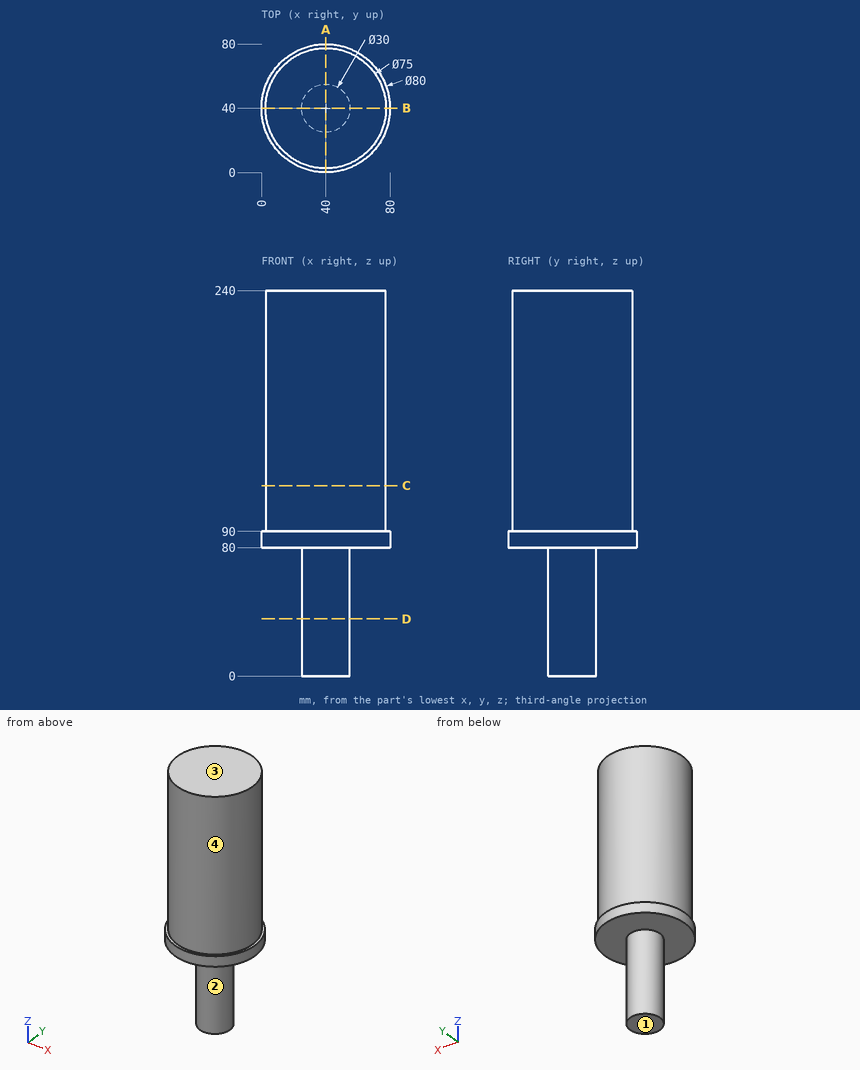
Geometry check sheet. Reference: drawing and pictorial views, mm from the part's lowest x, y, z. A direction names the side the tool comes from. Round coordinates to 2 decimals unless told otherwise and drop trailing zeros. Write each loop counter-clockwise with the first axis right and the second up, starting at its lowest first coordinate (ties: lowest second). Pieces come first, ordered by that corner, then holes.
(1) Section check D-D (z = 35.5). Enter the section's corners in (x, y), plus the area to 3 significant figures.
Returned:
outline: circle Ø30 at (40, 40)
area: 707 mm2
(2) Material ranges on line 1 (Z direction, x = 10, y = 33.5); line 2 (Y direction, x = 41.5, z = 188.5); line 3 (Z direction, x = 63, y = 9.5), recorded low to high.
Returned:
line 1: z = 80 to 240
line 2: y = 2.53 to 77.47
line 3: z = 80 to 90
(3) Section check A-A (x = 40). Enter the section's corners in (y, z), plus the area to 4 significant figures.
Returned:
outline: (0, 80) - (25, 80) - (25, 0) - (55, 0) - (55, 80) - (80, 80) - (80, 90) - (77.5, 90) - (77.5, 240) - (2.5, 240) - (2.5, 90) - (0, 90) - close
area: 14,450 mm2
(4) Mould release check, pull along Y, two halves, no side actions. Record for the marked faces 3 and 4: pulls with the +Y half, pulls with the -Y half, needs draft (parallel to the pull), parting line crosses it, or undercut.
Returned:
face 3: needs draft
face 4: parting line crosses it
(5) Section check C-C (z = 118.5). Enter the section's corners in (x, y), plus the area to 3 significant figures.
Returned:
outline: circle Ø75 at (40, 40)
area: 4,420 mm2
(6) Access from +Z, -Z, +X, -X, +Y, -Y to the whole of each face (thin tool, end or side, straight path). Record for the marked faces 1 and 2.
Returned:
face 1: -Z, +X, -X, +Y, -Y
face 2: -Z
(7) Depth check by flat-ended pin: pin 1 Ø6 at (y, z) = (23, 109) entering from -X; pin 2 Ø1.5 at (y, z) = (44.5, 96.5) entering from -X; pin 3 Ø1.5 at (x, z) = (42, 128.5) entering from -Y. Enter the tip coordinate at first touch or a pass-through.
Returned:
pin 1: stops at x = 5.21
pin 2: stops at x = 2.69
pin 3: stops at y = 2.52
